Here's how the part is built. I have some questions about the finished solid (model axes, mm). Face numbers are marked on the shaded views. A direction names the side the tool comes from. Round coordinates to 2 decimals unless told otherwise and drop trailing zeros. Write each loop counter-clockwise with the first axis right and the second up, starting at its lowest first coordinate (ties: lowest second). Pieces come first, ordered by that corner, then holes. Notation, with made-up numbers: (-23.75, 16) - (10.25, 16) arc R22 ccw to (10.25, 48) - close; hole circle Ø7 at (-31.5, 0.25). An arc over 180 degrees is marked (long way). Return JSON: item names as keys, results as strings. Group by question number.
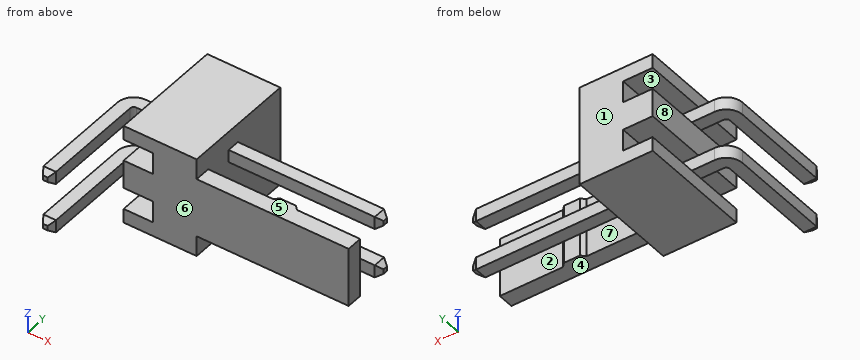
```python
from build123d import *
from OCP.BRepFilletAPI import BRepFilletAPI_MakeChamfer

# Parameters (mm, degrees)
SKETCH_1_W                           = 5.08
SKETCH_1_H                           = 5.8
EXTRUDE_1_DEPTH                      = 3.7
CUT_EXTRUDE_1_REACH                  = 9.334
SKETCH_5_W                           = 1.5
SKETCH_5_H                           = 1.1
EXTRUDE_START                        = 1.27
EXTRUDE_1_2_DEPTH                    = 0.32
CHAMFER_1_SIZE                       = 0.2
CHAMFER_1_SIZE2                      = 0.3
CHAMFER_2_SIZE                       = 0.3
CHAMFER_2_SIZE_2                     = 0.2
EXTRUDE_2_DEPTH                      = 1.5
PATTERN_LINEAR_2_COUNT               = 2
PATTERN_LINEAR_2_PITCH               = 2.54
CHAMFER_1_OF_PATTERN_LINEAR_2_SIZE2  = 0.2
CHAMFER_1_OF_PATTERN_LINEAR_2_SIZE   = 0.3
CHAMFER_2_OF_PATTERN_LINEAR_2_SIZE   = 0.3
CHAMFER_2_OF_PATTERN_LINEAR_2_SIZE_2 = 0.2


with BuildPart() as part:
    # Эскиз1 → Extrude 1 (new body)
    with BuildSketch(Plane(origin=(0, 0, 0), x_dir=(0, 0, -1), z_dir=(1, 0, 0))):
        with Locations((0, 2.9)):
            Rectangle(SKETCH_1_W, SKETCH_1_H)
    extrude(amount=EXTRUDE_1_DEPTH)

    # Эскиз5 → Вырез-Вытянуть1 (cut, up to next)
    with BuildSketch(Plane(origin=(0, 5.8, 0), x_dir=(1, 0, 0), z_dir=(0, 1, 0)), mode=Mode.PRIVATE) as cut_extrude_1_sk1:
        with Locations((0.75, -1.27)):
            Rectangle(SKETCH_5_W, SKETCH_5_H)
    cut_extrude_1_tool1 = extrude(cut_extrude_1_sk1.sketch, amount=-CUT_EXTRUDE_1_REACH, mode=Mode.PRIVATE) & part.part
    cut_extrude_1 = cut_extrude_1_tool1.solids().sort_by_distance((0.75, 5.8, 1.27))[0]
    add(cut_extrude_1, mode=Mode.SUBTRACT)

    # Эскиз3 → Extrude 1 2 (add, symmetric)
    with BuildSketch(Plane.XY.offset(EXTRUDE_START)):
        with BuildLine():
            Line((-1.16, -3.4), (-1.16, 2.04))
            ThreePointArc((-1.16, 2.04), (-1.107279221, 2.167279221), (-0.98, 2.22))
            Line((-0.98, 2.22), (11.4, 2.22))
            Line((11.4, 2.22), (11.4, 2.86))
            Line((11.4, 2.86), (-0.98, 2.86))
            ThreePointArc((-0.98, 2.86), (-1.559827561, 2.619827561), (-1.8, 2.04))
            Line((-1.8, 2.04), (-1.8, -3.4))
            Line((-1.8, -3.4), (-1.16, -3.4))
        make_face()
    extrude_1_2 = extrude(amount=EXTRUDE_1_2_DEPTH, both=True)

    # Фаска1
    chamfer_1_edges = [part.edges().sort_by_distance(p)[0] for p in [
        (11.4, 2.54, 1.59),
        (11.4, 2.22, 1.27),
        (11.4, 2.86, 1.27),
        (11.4, 2.54, 0.95),
    ]]
    chamfer_1_side = [part.faces().sort_by_distance(p)[0] for p in [
        (11.4, 2.54, 1.27),
    ]]
    chamfer(chamfer_1_edges, length=CHAMFER_1_SIZE, length2=CHAMFER_1_SIZE2, reference=chamfer_1_side[0])

    # Фаска2
    chamfer_2_edges_1 = [part.edges().sort_by_distance(p)[0] for p in [
        (-1.48, -3.4, 0.95),
    ]]
    chamfer_2_side_1 = [part.faces().sort_by_distance(p)[0] for p in [
        (-1.48, -3.396, 0.95),
    ]]
    chamfer_2_edges_2 = [part.edges().sort_by_distance(p)[0] for p in [
        (-1.48, -3.4, 1.59),
    ]]
    chamfer_2_side_2 = [part.faces().sort_by_distance(p)[0] for p in [
        (-1.48, -3.396, 1.59),
    ]]
    chamfer_2_edges_3 = [part.edges().sort_by_distance(p)[0] for p in [
        (-1.8, -3.4, 1.27),
    ]]
    chamfer_2_side_3 = [part.faces().sort_by_distance(p)[0] for p in [
        (-1.796, -3.4, 1.27),
    ]]
    chamfer_2_edges_4 = [part.edges().sort_by_distance(p)[0] for p in [
        (-1.16, -3.4, 1.27),
    ]]
    chamfer_2_side_4 = [part.faces().sort_by_distance(p)[0] for p in [
        (-1.16, -3.396, 1.27),
    ]]
    chamfer_2 = BRepFilletAPI_MakeChamfer(part.part.solid().wrapped)
    for e in chamfer_2_edges_1:
        chamfer_2.Add(CHAMFER_2_SIZE - 0.0001, CHAMFER_2_SIZE_2 - 0.0001, e.wrapped, chamfer_2_side_1[0].wrapped)
    for e in chamfer_2_edges_2:
        chamfer_2.Add(CHAMFER_2_SIZE - 0.0001, CHAMFER_2_SIZE_2 - 0.0001, e.wrapped, chamfer_2_side_2[0].wrapped)
    for e in chamfer_2_edges_3:
        chamfer_2.Add(CHAMFER_2_SIZE_2 - 0.0001, CHAMFER_2_SIZE - 0.0001, e.wrapped, chamfer_2_side_3[0].wrapped)
    for e in chamfer_2_edges_4:
        chamfer_2.Add(CHAMFER_2_SIZE - 0.0001, CHAMFER_2_SIZE_2 - 0.0001, e.wrapped, chamfer_2_side_4[0].wrapped)
    add(Compound.cast(chamfer_2.Shape()), mode=Mode.REPLACE)  # a hair under: the kernel refuses the full size

    # Эскиз4 → Бобышка-Вытянуть2 (add, symmetric)
    with BuildSketch(Plane.XY):
        Polygon((3.7, 0), (3.7, 0.8), (7, 0.8), (7.2, 1), (8, 1), (8.2, 0.8), (11.4, 0.8), (11.4, 0), align=None)
    extrude(amount=EXTRUDE_2_DEPTH, both=True)

    # Линейный массив2: Вырез-Вытянуть1, Extrude 1 2 ×2
    with Locations(*[(0, 0, -i * PATTERN_LINEAR_2_PITCH) for i in range(1, PATTERN_LINEAR_2_COUNT)]):
        add(cut_extrude_1, mode=Mode.SUBTRACT)
        add(extrude_1_2)

    # Фаска1 of Линейный массив2
    chamfer_1_of_pattern_linear_2_edges = [part.edges().sort_by_distance(p)[0] for p in [
        (11.4, 2.54, -0.95),
        (11.4, 2.22, -1.27),
        (11.4, 2.86, -1.27),
        (11.4, 2.54, -1.59),
    ]]
    chamfer(chamfer_1_of_pattern_linear_2_edges, length=CHAMFER_1_OF_PATTERN_LINEAR_2_SIZE, length2=CHAMFER_1_OF_PATTERN_LINEAR_2_SIZE2)

    # Фаска2 of Линейный массив2
    chamfer_2_of_pattern_linear_2_edges_1 = [part.edges().sort_by_distance(p)[0] for p in [
        (-1.48, -3.4, -1.59),
    ]]
    chamfer_2_of_pattern_linear_2_side_1 = [part.faces().sort_by_distance(p)[0] for p in [
        (-1.48, -3.396, -1.59),
    ]]
    chamfer_2_of_pattern_linear_2_edges_2 = [part.edges().sort_by_distance(p)[0] for p in [
        (-1.48, -3.4, -0.95),
    ]]
    chamfer_2_of_pattern_linear_2_side_2 = [part.faces().sort_by_distance(p)[0] for p in [
        (-1.48, -3.396, -0.95),
    ]]
    chamfer_2_of_pattern_linear_2_edges_3 = [part.edges().sort_by_distance(p)[0] for p in [
        (-1.8, -3.4, -1.27),
    ]]
    chamfer_2_of_pattern_linear_2_side_3 = [part.faces().sort_by_distance(p)[0] for p in [
        (-1.796, -3.4, -1.27),
    ]]
    chamfer_2_of_pattern_linear_2_edges_4 = [part.edges().sort_by_distance(p)[0] for p in [
        (-1.16, -3.4, -1.27),
    ]]
    chamfer_2_of_pattern_linear_2_side_4 = [part.faces().sort_by_distance(p)[0] for p in [
        (-1.16, -3.396, -1.27),
    ]]
    chamfer_2_of_pattern_linear_2 = BRepFilletAPI_MakeChamfer(part.part.solid().wrapped)
    for e in chamfer_2_of_pattern_linear_2_edges_1:
        chamfer_2_of_pattern_linear_2.Add(CHAMFER_2_OF_PATTERN_LINEAR_2_SIZE - 0.0001, CHAMFER_2_OF_PATTERN_LINEAR_2_SIZE_2 - 0.0001, e.wrapped, chamfer_2_of_pattern_linear_2_side_1[0].wrapped)
    for e in chamfer_2_of_pattern_linear_2_edges_2:
        chamfer_2_of_pattern_linear_2.Add(CHAMFER_2_OF_PATTERN_LINEAR_2_SIZE - 0.0001, CHAMFER_2_OF_PATTERN_LINEAR_2_SIZE_2 - 0.0001, e.wrapped, chamfer_2_of_pattern_linear_2_side_2[0].wrapped)
    for e in chamfer_2_of_pattern_linear_2_edges_3:
        chamfer_2_of_pattern_linear_2.Add(CHAMFER_2_OF_PATTERN_LINEAR_2_SIZE_2 - 0.0001, CHAMFER_2_OF_PATTERN_LINEAR_2_SIZE - 0.0001, e.wrapped, chamfer_2_of_pattern_linear_2_side_3[0].wrapped)
    for e in chamfer_2_of_pattern_linear_2_edges_4:
        chamfer_2_of_pattern_linear_2.Add(CHAMFER_2_OF_PATTERN_LINEAR_2_SIZE - 0.0001, CHAMFER_2_OF_PATTERN_LINEAR_2_SIZE_2 - 0.0001, e.wrapped, chamfer_2_of_pattern_linear_2_side_4[0].wrapped)
    add(Compound.cast(chamfer_2_of_pattern_linear_2.Shape()), mode=Mode.REPLACE)  # a hair under: the kernel refuses the full size


solid = part.part
```
1) For the marked faces 1, 2, 3, 4 and 5, which set-ups out of +Z, -Z, +X, -X, +Y, -Y let a thin tool reach every point of the face, with its end or its side?
2) Imagine slicing it at B-B (x = -0.75). Please give me the cut outline in (y, z).
3) Imagine slicing it at D-D (y = 1.25). Please give me the cut outline in (x, z).
4) Imagine slicing it at C-C (x = 4.75). Please give me the cut outline in (y, z), plus the area to 3 significant figures.
5) I need wall thicknesses on line 1 along Z through (x, y) = (5, 2.5); line 2 along X through (y, z) = (3.5, 1.7); line 3 along X through (y, z) = (4.25, -2.2). Which ranges of each line are inside material? Lowest first, please.
6) Will these pins go through, and if not, where does the flat tip stop? pin 1 Ø1.2 at (y, z) = (4, 1) entering from -X; pin 2 Ø0.5 at (x, z) = (7, 1.5) entering from +Y; pin 3 Ø0.9 at (x, z) = (5, 0) entering from +Y.
7) Imagine slicing it at A-A (y = -1). Please give me the cut outline in (x, z).
8) If we mould it in two halves opening along X, with no side actions, what happens to the marked faces 6, 7 and 8? For each: released by +X, released by -X, zero draft, split by the parting line, or undercut.
Results found:
{
 "1": {"face 1": "+Z, -Z, +X, -X, +Y", "face 2": "+Z, -Z, +X", "face 3": "-X, +Y, -Y", "face 4": "-Z, +X, -Y", "face 5": "+Z, +X, -Y"},
 "2": {"outline": "(2.22, -1.59) - (2.86, -1.59) - (2.86, -0.95) - (2.22, -0.95) - close; (2.22, 0.95) - (2.86, 0.95) - (2.86, 1.59) - (2.22, 1.59) - close"},
 "3": {"outline": "(-1.8, -1.59) - (-1.16, -1.59) - (-1.16, -0.95) - (-1.8, -0.95) - close; (-1.8, 0.95) - (-1.16, 0.95) - (-1.16, 1.59) - (-1.8, 1.59) - close; (0, -2.54) - (3.7, -2.54) - (3.7, 2.54) - (0, 2.54) - (0, 1.82) - (1.5, 1.82) - (1.5, 0.72) - (0, 0.72) - (0, -0.72) - (1.5, -0.72) - (1.5, -1.82) - (0, -1.82) - close"},
 "4": {"outline": "(0, -1.5) - (0.8, -1.5) - (0.8, 1.5) - (0, 1.5) - close; (2.22, -1.59) - (2.86, -1.59) - (2.86, -0.95) - (2.22, -0.95) - close; (2.22, 0.95) - (2.86, 0.95) - (2.86, 1.59) - (2.22, 1.59) - close", "area": "3.22 mm²"},
 "5": {"line 1": "z = -1.59 to -0.95, 0.95 to 1.59", "line 2": "x = 1.5 to 3.7", "line 3": "x = 0 to 3.7"},
 "6": {"pin 1": "stops at x = 0", "pin 2": "stops at y = 2.86", "pin 3": "stops at y = 0.8"},
 "7": {"outline": "(-1.8, -1.59) - (-1.16, -1.59) - (-1.16, -0.95) - (-1.8, -0.95) - close; (-1.8, 0.95) - (-1.16, 0.95) - (-1.16, 1.59) - (-1.8, 1.59) - close"},
 "8": {"face 6": "zero draft", "face 7": "undercut", "face 8": "released by -X"}
}
